from build123d import *

# Parameters (mm, degrees)
SKETCH_1_W          = 88.3
SKETCH_1_H          = 59.7
SKETCH_1_W_2        = 82.3
SKETCH_1_H_2        = 53.7
EXTRUDE_1_DEPTH     = 8
SKETCH_2_W          = 88.3
SKETCH_2_H          = 59.7
EXTRUDE_2_DEPTH     = 2
SKETCH_3_W          = 59.09959803
SKETCH_3_H          = 34.490013092
CUT_EXTRUDE_1_DEPTH = 2
SKETCH_4_W          = 3
SKETCH_4_H          = 53.7
CUT_EXTRUDE_2_DEPTH = 8
SKETCH_5_W          = 11
SKETCH_5_H          = 3
CUT_EXTRUDE_3_DEPTH = 6
SKETCH_6_W          = 1.375438735
SKETCH_6_H          = 2
EXTRUDE_3_DEPTH     = 11
EXTRUDE_4_REACH     = 62.49
SKETCH_7_W          = 1.5
SKETCH_7_H          = 2


with BuildPart() as part:
    # 草图1 → 凸台-拉伸1 (new body)
    with BuildSketch(Plane(origin=(0, 0, 0), x_dir=(1, 0, 0), z_dir=(0, 1, 0))):
        Rectangle(SKETCH_1_W, SKETCH_1_H)
        Rectangle(SKETCH_1_W_2, SKETCH_1_H_2, mode=Mode.SUBTRACT)
    extrude(amount=EXTRUDE_1_DEPTH)

    # 草图2 → 凸台-拉伸2 (add)
    with BuildSketch(Plane.XZ):
        Rectangle(SKETCH_2_W, SKETCH_2_H)
    extrude(amount=EXTRUDE_2_DEPTH)

    # 草图3 → 切除-拉伸1 (cut)
    with BuildSketch(Plane(origin=(0, 0, 0), x_dir=(1, 0, 0), z_dir=(0, 1, 0))):
        Rectangle(SKETCH_3_W, SKETCH_3_H)
    extrude(amount=-CUT_EXTRUDE_1_DEPTH, mode=Mode.SUBTRACT)

    # 草图4 → 切除-拉伸2 (cut)
    with BuildSketch(Plane(origin=(0, 8, 0), x_dir=(1, 0, 0), z_dir=(0, 1, 0))):
        with Locations((-42.65, 0)):
            Rectangle(SKETCH_4_W, SKETCH_4_H)
    extrude(amount=-CUT_EXTRUDE_2_DEPTH, mode=Mode.SUBTRACT)

    # 草图5 → 切除-拉伸3 (cut)
    with BuildSketch(Plane(origin=(0, 8, 0), x_dir=(1, 0, 0), z_dir=(0, 1, 0))):
        with Locations((-13.35, 28.35)):
            Rectangle(SKETCH_5_W, SKETCH_5_H)
        with Locations((-13.35, -28.35)):
            Rectangle(SKETCH_5_W, SKETCH_5_H)
    extrude(amount=-CUT_EXTRUDE_3_DEPTH, mode=Mode.SUBTRACT)

    # 草图6 → 凸台-拉伸3 (add)
    with BuildSketch(Plane.ZY.offset(7.85)):
        with Locations((29.162280632, 7)):
            Rectangle(SKETCH_6_W, SKETCH_6_H)
    extrude(amount=EXTRUDE_3_DEPTH)

    # 草图7 → 凸台-拉伸4 (add, up to next)
    with BuildSketch(Plane.ZY.offset(7.85), mode=Mode.PRIVATE) as extrude_4_sk1:
        with Locations((-29.1, 7)):
            Rectangle(SKETCH_7_W, SKETCH_7_H)
    extrude_4_tool1 = extrude(extrude_4_sk1.sketch, amount=EXTRUDE_4_REACH, mode=Mode.PRIVATE) - part.part
    add(extrude_4_tool1.solids().sort_by_distance((-7.85, 7, -29.1))[0])


solid = part.part
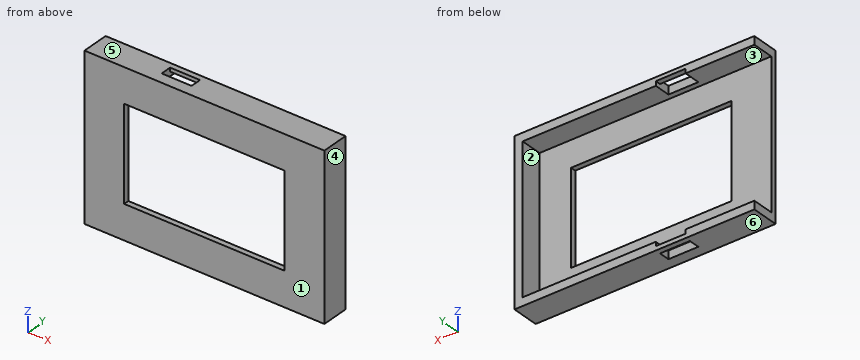
Can you work these out from the model? Positions are in its coordinate system, mm. Face numbers are marked on the shaded views. A direction names the side the tool comes from. Give positions to 0.01 mm unless a question says otherwise; leave off trailing zeros. Order: outer loops, then holes, each group sorted by start corner. A loop starts at its lowest first (then second) coordinate and runs counter-clockwise, first axis right, second up. Notation, with made-up numbers: M 27,-5 L 42,-5 A21 ccw 42,19 Z; hole C 7.5,2.25 d4. An arc over 180 degrees is marked long. Use one line per item in the form item = value. Start each with the question number.
Item 1: We'd pull the mould along Z, two halves only. Please class the marked faces 3, 4, 5 and 6: +Z half, -Z half, draft (parallel to the pull), parting line (faces both ways), or undercut.
Item 2: For the marked faces 1 and 2, which set-ups out of +Z, -Z, +X, -X, +Y, -Y let a thin tool reach every point of the face, with its end or its side?
Item 3: If we section it at D-D (x = -13): Write out the boundary of the cut face in (y, z) (3 decimals), then the cut area to 3 significant figures.
Item 4: Will these pins go through, and if not, where does the flat tip stop? pin 1 Ø1.5 at (y, z) = (6.5, -5.5) entering from -X; pin 2 Ø2 at (x, z) = (-21, -18.5) entering from +Y.
Item 5: If I drill on line 1 along Z through (x, y) = (-26, 4.5); line 2 along Z through (x, y) = (7, -1.25) (3 decimals); line 3 along X through (y, z) = (-0.5, 5.5), over which ranges is the centre line in solid material (lowest first)?
Item 6: If we section it at B-B (y = 5): Write out the boundary of the cut face in (x, z), then the cut area to 3 significant figures.
Item 7: If we section it at C-C (z = -11): Write out the boundary of the cut face in (x, y), then the cut area to 3 significant figures.
Item 8: If we section it at A-A (x = -26.5): Write out the boundary of the cut face in (y, z) (3 decimals), then the cut area to 3 significant figures.
Outcome:
q1.face_3 = undercut
q1.face_4 = draft
q1.face_5 = +Z half
q1.face_6 = -Z half
q2.face_1 = +Z, -Z, +X, -X, -Y
q2.face_2 = -X, +Y
q3.outline = M -2,-29.85 L 2,-29.85 L 2,-26.85 L 0,-26.85 L 0,-17.245 L -2,-17.245 Z; M -2,17.245 L 0,17.245 L 0,26.85 L 2,26.85 L 2,29.85 L -2,29.85 Z; M 6,-29.85 L 8,-29.85 L 8,-28.35 L 6,-28.35 Z; M 6,28.475 L 8,28.475 L 8,29.85 L 6,29.85 Z
q3.area = 68.2 mm2
q4.pin_1 = 41.15
q4.pin_2 = 0
q5.line_1 = -29.85 to -26.85, 26.85 to 29.85
q5.line_2 = -29.85 to -17.245, 17.245 to 29.85
q5.line_3 = -44.15 to -29.55, 29.55 to 44.15
q6.outline = M -44.15,-29.85 L -18.85,-29.85 L -18.85,-26.85 L -44.15,-26.85 Z; M -44.15,26.85 L -18.85,26.85 L -18.85,29.85 L -44.15,29.85 Z; M -7.85,-29.85 L 44.15,-29.85 L 44.15,29.85 L -7.85,29.85 L -7.85,26.85 L 41.15,26.85 L 41.15,-26.85 L -7.85,-26.85 Z
q6.area = 625 mm2
q7.outline = M -44.15,-2 L -29.55,-2 L -29.55,0 L -44.15,0 Z; M 29.55,-2 L 44.15,-2 L 44.15,8 L 41.15,8 L 41.15,0 L 29.55,0 Z
q7.area = 82.4 mm2
q8.outline = M -2,-29.85 L 8,-29.85 L 8,-26.85 L 0,-26.85 L 0,-17.245 L -2,-17.245 Z; M -2,17.245 L 0,17.245 L 0,26.85 L 8,26.85 L 8,29.85 L -2,29.85 Z
q8.area = 98.4 mm2
